Autodesk Inventor part; units mm, degrees
ref_plane "YZ Plane" through (0, 0, 0) normal (1, 0, 0) x (0, 1, 0)
ref_plane "XZ Plane" through (0, 0, 0) normal (0, 1, 0) x (-1, 0, 0)
ref_plane "XY Plane" through (0, 0, 0) normal (0, 0, 1) x (1, 0, 0)
sketch "Sketch1" plane through (0, 0, 0) normal (0, 1, 0) x (-1, 0, 0)
  point P0 (0, 0)
sketch "Sketch2" plane through (0, 0, 0) normal (0, 1, 0) x (-1, 0, 0)
  line L0 (-100, 100) -> (100, 100)
  line L1 (100, 100) -> (100, -100)
  line L2 (100, -100) -> (-100, -100)
  line L3 (-100, -100) -> (-100, 100)
  line L4 (-100, 100) -> (100, -100) construction
  line L5 (100, 100) -> (-100, -100) construction
  line L6 (95, 10) -> (75, 10)
  line L7 (75, 10) -> (75, -10)
  line L8 (75, -10) -> (95, -10)
  line L9 (95, -10) -> (95, 10)
  line L10 (95, 10) -> (75, -10) construction
  line L11 (75, 10) -> (95, -10) construction
  circle A0 centre (95, 10) radius 1.5
  circle A1 centre (95, -10) radius 1.5
  circle A2 centre (75, -10) radius 1.5
  circle A3 centre (75, 10) radius 1.5
  line L12 (-10, 95) -> (-10, 75)
  circle A4 centre (-10, 95) radius 1.5
  circle A5 centre (-10, 75) radius 1.5
  line L13 (-10, 75) -> (10, 75)
  line L14 (10, 75) -> (10, 95)
  line L15 (-10, 75) -> (10, 95) construction
  line L16 (-10, 95) -> (10, 75) construction
  line L17 (10, 95) -> (-10, 95)
  circle A6 centre (10, 95) radius 1.5
  circle A7 centre (10, 75) radius 1.5
  line L18 (-95, -10) -> (-75, -10)
  circle A8 centre (-95, -10) radius 1.5
  circle A9 centre (-75, -10) radius 1.5
  line L19 (-75, -10) -> (-75, 10)
  line L20 (-75, 10) -> (-95, 10)
  line L21 (-75, -10) -> (-95, 10) construction
  line L22 (-95, -10) -> (-75, 10) construction
  line L23 (-95, 10) -> (-95, -10)
  circle A10 centre (-95, 10) radius 1.5
  circle A11 centre (-75, 10) radius 1.5
  line L24 (10, -95) -> (10, -75)
  circle A12 centre (10, -95) radius 1.5
  circle A13 centre (10, -75) radius 1.5
  line L25 (10, -75) -> (-10, -75)
  line L26 (-10, -75) -> (-10, -95)
  line L27 (10, -75) -> (-10, -95) construction
  line L28 (10, -95) -> (-10, -75) construction
  line L29 (-10, -95) -> (10, -95)
  circle A14 centre (-10, -95) radius 1.5
  circle A15 centre (-10, -75) radius 1.5
  point P0 (0, 0)
  point P1 (85, 0)
  point P2 (0, 85)
  point P3 (-85, 0)
  point P4 (0, -85)
  dimension "d0" = 200
  dimension "d1" = 200
  dimension "d2" = 20
  dimension "d3" = 20
  dimension "d4" = 5
  dimension "d5" = 3
  dimension "d6" = 3
  dimension "d7" = 3
  dimension "d8" = 3
  dimension "d11" = 360
extrude "Extrusion1" add sketch "Sketch2" along normal blind 5.4 contours L0 L1 L2 L3 | L6 A0 L9 A1 L8 A2 L7 A3 | A4 L17 A6 L14 A7 L13 A5 L12 | A8 L23 A10 L20 A11 L19 A9 L18 | A12 L29 A14 L26 A15 L25 A13 L24
chamfer "Chamfer1" distance 20 angle 45 4 edges at (100, 2.7, -100) (-100, 2.7, -100) (100, 2.7, 100) (-100, 2.7, 100)
sketch "Sketch5" plane through (0, 0, 0) normal (0, -1, 0) x (1, 0, 0)
  circle A0 centre (0, 0) radius 4
  circle A1 centre (0, 0) radius 1.45
  dimension "d32" = 2.9
  dimension "d33" = 8
extrude "Extrusion3" cut sketch "Sketch5" against normal blind 8 contours A1
pattern_linear "Rectangular Pattern1" count 5 spacing 15 along (1, 0, 0) count 5 spacing 15 along (0, 0, 1) of "Extrusion3"
mirror "Mirror1" about plane through (0, 0, 0) normal (1, 0, 0) of "Extrusion3", "Rectangular Pattern1"
mirror "Mirror2" about plane through (0, 0, 0) normal (0, 0, 1) of "Extrusion3", "Rectangular Pattern1", "Mirror1"
sketch "Sketch6" plane through (0, 5.4, 0) normal (0, 1, 0) x (1, 0, 0)
  line L0 (-100, 80) -> (-80, 100)
  line L1 (-90, 90) -> (-75.8579, 75.8579)
  circle A0 centre (-75.8579, 75.8579) radius 1.5
  point P0 (0, 0)
  dimension "d44" = 3
  dimension "d45" = 20
extrude "Extrusion5" cut sketch "Sketch6" against normal blind 16
pattern_circular "Circular Pattern1" count 4 over 360 about axis through (0, 0, 0) along (0, 1, 0) of "Extrusion5"
sketch "Sketch8" plane through (0, 5.4, 0) normal (0, 1, 0) x (1, 0, 0)
  line L0 (46.45, -46.45) -> (-46.45, -46.45)
  line L1 (-46.45, -46.45) -> (-46.45, 46.45)
  line L2 (-46.45, 46.45) -> (46.45, 46.45)
  line L3 (46.45, 46.45) -> (46.45, -46.45)
  circle A0 centre (0, 0) radius 1.45
  line L4 (46.45, -46.45) -> (-46.45, 46.45) construction
  line L5 (-46.45, -46.45) -> (46.45, 46.45) construction
extrude "Extrusion7" cut sketch "Sketch8" against normal blind 10
equation "\"d34\" = d33"
properties part number "RobotBase"
Design review of the part built by this model. Coordinates are the model's own, in mm. A direction names the side the tool comes from. Round coordinates to 2 decimals unless told otherwise and drop trailing zeros. Order: outer loops, then holes, each group sorted by start corner. A loop starts at its lowest first (then second) coordinate and runs counter-clockwise, first axis right, second up. Notation, with made-up numbers: (81.5, -19) - (140.5, -19) arc R25 ccw to (140.5, -6) - close; hole circle Ø8 at (18.25, -24). An arc over 180 degrees is marked (long way). Return JSON: item names as keys, results as strings.
Q1. For pin 1 Ø4 at (x, z) = (60, -45) entering from +Y, flat-tipped, find the tip position at first contact; note if it passes through.
Computed values:
{"pin 1": "stops at y = 5.4"}
Q2. Consider section A-A on x = -4.5. Write out the cut boundary in (y, z).
Computed values:
{"outline": "(0, -100) - (5.4, -100) - (5.4, -46.45) - (0, -46.45) - close; (0, 46.45) - (5.4, 46.45) - (5.4, 100) - (0, 100) - close"}
Q3. Machinability: for faces 1 (the flat face through (-1, 3, -46.45)), 2 (the flat face through (-90, 3, 90)), which of the approach directions +Z, -Z, +X, -X, +Y, -Y give a long, thin tool a straight path to every point of the face, cutting with its end or side? Answer none if there is none.
Computed values:
{"face 1": "+Y, -Y", "face 2": "+Z, -X, +Y, -Y"}
Q4. Consider section B-B on z = 20.5. Write out the cut boundary in (x, y), plus the area to 3 significant figures.
Computed values:
{"outline": "(-100, 0) - (-46.45, 0) - (-46.45, 5.4) - (-100, 5.4) - close; (46.45, 0) - (100, 0) - (100, 5.4) - (46.45, 5.4) - close", "area": "578 mm2"}
Q5. Consider section C-C on x = 86. Write out the cut boundary in (y, z), plus the area to 3 significant figures.
Computed values:
{"outline": "(0, -94) - (5.4, -94) - (5.4, 94) - (0, 94) - close", "area": "1,020 mm2"}
Q6. Consider section D-D on y = 3.8. Give the number of separate pieces and of enclosed holes in the cut face, plus the area to 3 significant figures.
Computed values:
{"separate pieces": "1", "enclosed holes": "53", "area": "30,200 mm2"}
Q7. The part is to be moulded in two halves that separate along Z. For faces 3 (the flat face through (-46.45, 3, 1)), 4 (the flat face through (90, 3, -90)), 5 (the flat face through (1, 0, -65)), 6 (the flat face through (90, 3, 90)), say which applies: pulls with the +Z half, pulls with the -Z half, needs draft (parallel to the pull), parting line crosses it, or undercut.
Computed values:
{"face 3": "undercut", "face 4": "pulls with the -Z half", "face 5": "needs draft", "face 6": "pulls with the +Z half"}
Q8. Wall thickness on L1, parallel to X at y = 4.2, z = -45; L2, parallel to X at y = 1.35, z = -17: over which ranges is each line inside the solid? List them lowest first. Write a range as [from, to].
Computed values:
{"L1": "x = [-100, -61.45], [-58.55, -46.45], [46.45, 58.55], [61.45, 100]", "L2": "x = [-100, -46.45], [46.45, 100]"}
